Autodesk Inventor part; units mm, degrees
ref_plane "YZ Plane" through (0, 0, 0) normal (1, 0, 0) x (0, 1, 0)
ref_plane "XZ Plane" through (0, 0, 0) normal (0, 1, 0) x (-1, 0, 0)
ref_plane "XY Plane" through (0, 0, 0) normal (0, 0, 1) x (1, 0, 0)
sketch "スケッチ1" plane through (0, 0, 0) normal (0, 1, 0) x (-1, 0, 0)
  line L0 (0, 0) -> (40, 0)
  line L1 (40, 0) -> (40, 90)
  line L2 (40, 90) -> (0, 90)
  line L3 (0, 90) -> (0, 0)
  line L4 (0, 90) -> (10, 90)
  line L5 (10, 90) -> (10, 76.25)
  line L6 (10, 75) -> (0, 75)
  line L7 (0, 75) -> (0, 90)
  line L8 (40, 90) -> (30, 90)
  line L9 (30, 90) -> (30, 76.25)
  line L10 (30, 75) -> (40, 75)
  line L11 (40, 75) -> (40, 90)
  line L12 (0, 0) -> (10, 0)
  line L13 (10, 0) -> (10, 13.75)
  line L14 (10, 15) -> (0, 15)
  line L15 (0, 15) -> (0, 0)
  line L16 (40, 0) -> (30, 0)
  line L17 (30, 0) -> (30, 13.75)
  line L18 (30, 15) -> (40, 15)
  line L19 (40, 15) -> (40, 0)
  circle A0 centre (10, 75) radius 1.25
  circle A1 centre (30, 75) radius 1.25
  circle A2 centre (10, 45) radius 1.25
  circle A3 centre (30, 45) radius 1.25
  circle A4 centre (10, 15) radius 1.25
  circle A5 centre (30, 15) radius 1.25
  dimension "d10" = 2.5
  dimension "d11" = 2.5
  dimension "d14" = 2.5
  dimension "d15" = 2.5
  dimension "d0" = 40
  dimension "d1" = 90
  dimension "d2" = 10
  dimension "d3" = 15
  dimension "d4" = 10
  dimension "d5" = 15
  dimension "d6" = 10
  dimension "d7" = 15
  dimension "d8" = 10
  dimension "d9" = 15
  dimension "d12" = 2.5
  dimension "d13" = 2.5
extrude "押し出し1" add sketch "スケッチ1" along normal blind 19.7 contours L3 L14 A4 L13 L0 | L13 A4 L14 L3 L6 A0 L5 L2 L9 A1 L10 L1 L18 A5 L17 L0 | L17 A5 L18 L1 L0 | L3 L2 L5 A0 L6 | L10 A1 L9 L2 L1
properties part number "知能ロボコンスペーサ1.1"
Verification items for the finished model (mm, model axes). Round coordinates to 2 decimals unless told otherwise and drop trailing zeros. Write each loop counter-clockwise with the first axis right and the second up, starting at its lowest first coordinate (ties: lowest second). Pieces come first, ordered by that corner, then holes. Notation, with made-up numbers: (19, -10.5) -> (32, -10.5) arc R22 ccw to (32, 14.5) -> close; hole circle Ø11 at (11, 40.5). An arc over 180 degrees is marked (long way). Write each question's results on one line, items separated by ' | '.
Q1. Sectioned sample at B-B, the plane z = 75. Record the boundary of the cut face in (x, y).
Derived:
outline: (-40, 0) -> (-31.25, 0) -> (-31.25, 19.7) -> (-40, 19.7) -> close; (-28.75, 0) -> (-11.25, 0) -> (-11.25, 19.7) -> (-28.75, 19.7) -> close; (-8.75, 0) -> (0, 0) -> (0, 19.7) -> (-8.75, 19.7) -> close
Q2. Thickness scan on probe 1 along Z at (x, y) = (-10, 11.75); probe 2 along X at (y, z) = (7.5, 15); probe 3 along Z at (x, y) = (-9, 13.5). Record the ranges inside material, lowest first.
Derived:
probe 1: z = 0 to 13.75, 16.25 to 43.75, 46.25 to 73.75, 76.25 to 90 | probe 2: x = -40 to -31.25, -28.75 to -11.25, -8.75 to 0 | probe 3: z = 0 to 14.25, 15.75 to 44.25, 45.75 to 74.25, 75.75 to 90
Q3. Draft check along X on faces 1 (the face through (-40, 10, 44)), 2 (the face through (-20, 19.7, 46)), 3 (the face through (-9.84, 9.71, 73.76)). Enter one of: released by +X, released by -X, zero draft, split by the parting line, or undercut.
Derived:
face 1: released by -X | face 2: zero draft | face 3: undercut
Q4. Sectioned sample at A-A, the plane x = -10. Record the boundary of the cut face in (y, z).
Derived:
outline: (0, 0) -> (19.7, 0) -> (19.7, 13.75) -> (0, 13.75) -> close; (0, 16.25) -> (19.7, 16.25) -> (19.7, 43.75) -> (0, 43.75) -> close; (0, 46.25) -> (19.7, 46.25) -> (19.7, 73.75) -> (0, 73.75) -> close; (0, 76.25) -> (19.7, 76.25) -> (19.7, 90) -> (0, 90) -> close
